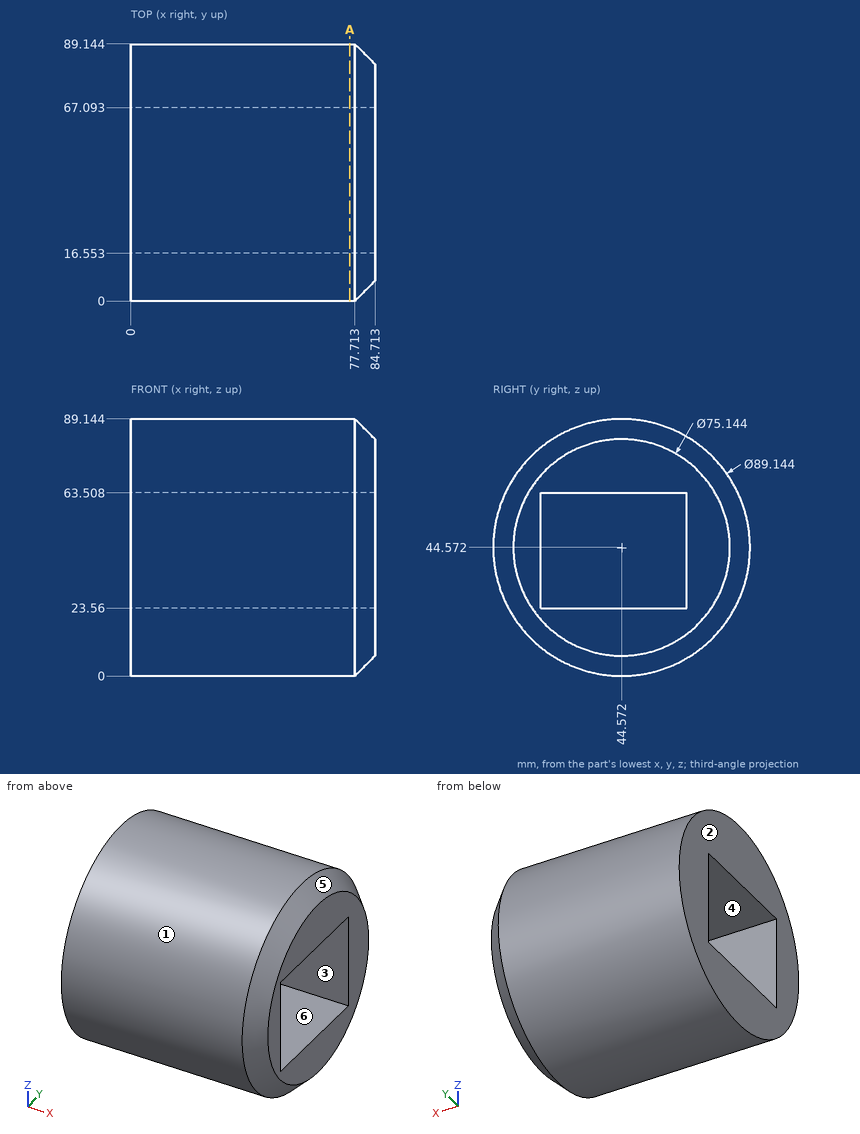
Design review of the part shown in the three views and the two pictorial views. Dimensions are in mm from the part's minimum x, y and z. A direction names the side the tool comes from. Coordinates: 2 decimals unless noted, no trailing zeros. Write each loop counter-clockwise with the first axis right and the second up, starting at its lowest first coordinate (ties: lowest second). Pieces come first, ordered by that corner, then holes. Notation, with made-up numbers: (-30, 34.25) - (-15, 34.25) arc R15 cw to (-15, 46.25) - close; hole circle Ø4 at (70.25, 64.25). An arc over 180 degrees is marked (long way). Write item = value, one per line.
(1) Mouldability with a two-part tool opening along Z and no side actions: class the marked faces 1, 2, 3 and 4 as pulls with the +Z half, pulls with the -Z half, needs draft (parallel to the pull), parting line crosses it, or undercut.
Result sheet:
face_1 = parting line crosses it
face_2 = needs draft
face_3 = undercut
face_4 = undercut
(2) For P1, Ø5, axis at x = 12, y = 67.5, coming from the -Z side; P2, Ø2, axis at y = 15, z = 18.5, coming from the +X side; P3, Ø6, axis at x = 30, y = 73.5, coming from the +Z side, all flat-tipped, find the tip position at first contact; note any pin that passes through.
Result sheet:
P1 = 4.96
P2 = 83.86
P3 = 80.83
(3) Consider section A-A, the plane x = 76. Give the boundary of the cut face in (y, z).
Result sheet:
outline = circle Ø89.14 at (44.57, 44.57); hole (16.55, 23.56) - (67.09, 23.56) - (67.09, 63.51) - (16.55, 63.51) - close
(4) Machinability: for the marked faces 5 and 6, which of the approach directions +Z, -Z, +X, -X, +Y, -Y give a long, thin tool a straight path to every point of the face, cutting with its end or side? Answer none if there is none.
Result sheet:
face_5 = +X
face_6 = +X, -X
(5) For line 1 (Z direction, x = 61.5, y = 46); line 2 (Z direction, x = 31, y = 30.5) (1 decimal); line 3 (Y direction, x = 31, z = 25), list the stretches that pass through material, from the lowest coordinate up. Write a range as [from, to].
Result sheet:
line_1 = [0.02, 23.56], [63.51, 89.12]
line_2 = [2.3, 23.6], [63.5, 86.9]
line_3 = [4.53, 16.55], [67.09, 84.62]
